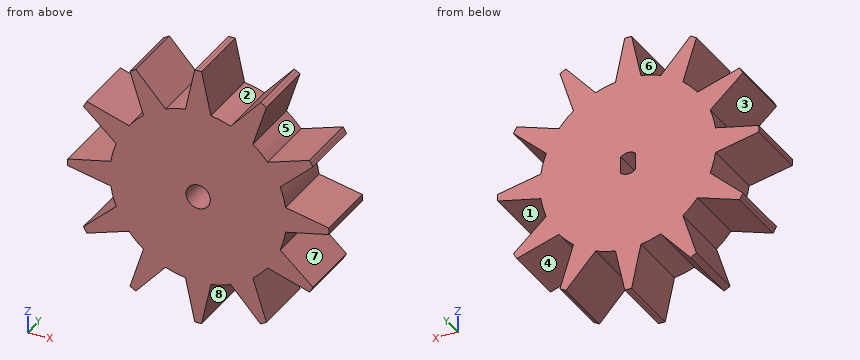
from build123d import *

# Parameters (mm, degrees)
F1_DEPTH = 17.5
F3_DEPTH = 9
F4_R     = 3.25
F5_DEPTH = 9


with BuildPart() as f1:
    # F0 (on Front) → F1 (new body)
    with BuildSketch(Plane.XZ):
        with BuildLine():
            ThreePointArc((23.401412, -3.42), (23.587771, -1.714511), (23.65, 0))
            ThreePointArc((23.65, 0), (23.587771, 1.714511), (23.401412, 3.42))
            ThreePointArc((23.401412, 3.42), (22.844146, 6.12107), (21.976218, 8.738899))
            ThreePointArc((21.976218, 8.738899), (20.481501, 11.825), (18.556218, 14.662513))
            ThreePointArc((18.556218, 14.662513), (16.723075, 16.723075), (14.662513, 18.556218))
            ThreePointArc((14.662513, 18.556218), (11.825, 20.481501), (8.738899, 21.976218))
            ThreePointArc((8.738899, 21.976218), (6.12107, 22.844146), (3.42, 23.401412))
            ThreePointArc((3.42, 23.401412), (0, 23.65), (-3.42, 23.401412))
            ThreePointArc((-3.42, 23.401412), (-6.12107, 22.844146), (-8.738899, 21.976218))
            ThreePointArc((-8.738899, 21.976218), (-11.825, 20.481501), (-14.662513, 18.556218))
            ThreePointArc((-14.662513, 18.556218), (-16.723075, 16.723075), (-18.556218, 14.662513))
            ThreePointArc((-18.556218, 14.662513), (-20.481501, 11.825), (-21.976218, 8.738899))
            ThreePointArc((-21.976218, 8.738899), (-22.844146, 6.12107), (-23.401412, 3.42))
            ThreePointArc((-23.401412, 3.42), (-23.65, 0), (-23.401412, -3.42))
            ThreePointArc((-23.401412, -3.42), (-22.844146, -6.12107), (-21.976218, -8.738899))
            ThreePointArc((-21.976218, -8.738899), (-20.481501, -11.825), (-18.556218, -14.662513))
            ThreePointArc((-18.556218, -14.662513), (-16.723075, -16.723075), (-14.662513, -18.556218))
            ThreePointArc((-14.662513, -18.556218), (-11.825, -20.481501), (-8.738899, -21.976218))
            ThreePointArc((-8.738899, -21.976218), (-6.12107, -22.844146), (-3.42, -23.401412))
            ThreePointArc((-3.42, -23.401412), (0, -23.65), (3.42, -23.401412))
            ThreePointArc((3.42, -23.401412), (6.12107, -22.844146), (8.738899, -21.976218))
            ThreePointArc((8.738899, -21.976218), (11.825, -20.481501), (14.662513, -18.556218))
            ThreePointArc((14.662513, -18.556218), (16.723075, -16.723075), (18.556218, -14.662513))
            ThreePointArc((18.556218, -14.662513), (20.481501, -11.825), (21.976218, -8.738899))
            ThreePointArc((21.976218, -8.738899), (22.844146, -6.12107), (23.401412, -3.42))
        make_face()
        with BuildLine():
            ThreePointArc((23.401412, 3.42), (23.587771, 1.714511), (23.65, 0))
            ThreePointArc((23.65, 0), (23.587771, -1.714511), (23.401412, -3.42))
            Line((23.401412, -3.42), (34.98804, -0.914922))
            Line((34.98804, -0.914922), (35, 0))
            Line((35, 0), (34.98804, 0.914922))
            Line((34.98804, 0.914922), (23.401412, 3.42))
        make_face()
        with BuildLine():
            ThreePointArc((18.556218, 14.662513), (20.481501, 11.825), (21.976218, 8.738899))
            Line((21.976218, 8.738899), (30.757992, 16.701674))
            Line((30.757992, 16.701674), (30.310889, 17.5))
            Line((30.310889, 17.5), (29.84307, 18.286365))
            Line((29.84307, 18.286365), (18.556218, 14.662513))
        make_face()
        with BuildLine():
            Line((30.757992, -16.701674), (21.976218, -8.738899))
            ThreePointArc((21.976218, -8.738899), (20.481501, -11.825), (18.556218, -14.662513))
            Line((18.556218, -14.662513), (29.84307, -18.286365))
            Line((29.84307, -18.286365), (30.310889, -17.5))
            Line((30.310889, -17.5), (30.757992, -16.701674))
        make_face()
        with BuildLine():
            ThreePointArc((8.738899, 21.976218), (11.825, 20.481501), (14.662513, 18.556218))
            Line((14.662513, 18.556218), (18.286365, 29.84307))
            Line((18.286365, 29.84307), (17.5, 30.310889))
            Line((17.5, 30.310889), (16.701674, 30.757992))
            Line((16.701674, 30.757992), (8.738899, 21.976218))
        make_face()
        with BuildLine():
            Line((18.286365, -29.84307), (14.662513, -18.556218))
            ThreePointArc((14.662513, -18.556218), (11.825, -20.481501), (8.738899, -21.976218))
            Line((8.738899, -21.976218), (16.701674, -30.757992))
            Line((16.701674, -30.757992), (17.5, -30.310889))
            Line((17.5, -30.310889), (18.286365, -29.84307))
        make_face()
        with BuildLine():
            ThreePointArc((-3.42, 23.401412), (0, 23.65), (3.42, 23.401412))
            Line((3.42, 23.401412), (0.914922, 34.98804))
            Line((0.914922, 34.98804), (0, 35))
            Line((0, 35), (-0.914922, 34.98804))
            Line((-0.914922, 34.98804), (-3.42, 23.401412))
        make_face()
        with BuildLine():
            Line((0.914922, -34.98804), (3.42, -23.401412))
            ThreePointArc((3.42, -23.401412), (0, -23.65), (-3.42, -23.401412))
            Line((-3.42, -23.401412), (-0.914922, -34.98804))
            Line((-0.914922, -34.98804), (0, -35))
            Line((0, -35), (0.914922, -34.98804))
        make_face()
        with BuildLine():
            ThreePointArc((-14.662513, 18.556218), (-11.825, 20.481501), (-8.738899, 21.976218))
            Line((-8.738899, 21.976218), (-16.701674, 30.757992))
            Line((-16.701674, 30.757992), (-17.5, 30.310889))
            Line((-17.5, 30.310889), (-18.286365, 29.84307))
            Line((-18.286365, 29.84307), (-14.662513, 18.556218))
        make_face()
        with BuildLine():
            Line((-16.701674, -30.757992), (-8.738899, -21.976218))
            ThreePointArc((-8.738899, -21.976218), (-11.825, -20.481501), (-14.662513, -18.556218))
            Line((-14.662513, -18.556218), (-18.286365, -29.84307))
            Line((-18.286365, -29.84307), (-17.5, -30.310889))
            Line((-17.5, -30.310889), (-16.701674, -30.757992))
        make_face()
        with BuildLine():
            ThreePointArc((-21.976218, 8.738899), (-20.481501, 11.825), (-18.556218, 14.662513))
            Line((-18.556218, 14.662513), (-29.84307, 18.286365))
            Line((-29.84307, 18.286365), (-30.310889, 17.5))
            Line((-30.310889, 17.5), (-30.757992, 16.701674))
            Line((-30.757992, 16.701674), (-21.976218, 8.738899))
        make_face()
        with BuildLine():
            Line((-29.84307, -18.286365), (-18.556218, -14.662513))
            ThreePointArc((-18.556218, -14.662513), (-20.481501, -11.825), (-21.976218, -8.738899))
            Line((-21.976218, -8.738899), (-30.757992, -16.701674))
            Line((-30.757992, -16.701674), (-30.310889, -17.5))
            Line((-30.310889, -17.5), (-29.84307, -18.286365))
        make_face()
        with BuildLine():
            ThreePointArc((-23.401412, -3.42), (-23.65, 0), (-23.401412, 3.42))
            Line((-23.401412, 3.42), (-34.98804, 0.914922))
            Line((-34.98804, 0.914922), (-35, 0))
            Line((-35, 0), (-34.98804, -0.914922))
            Line((-34.98804, -0.914922), (-23.401412, -3.42))
        make_face()
    extrude(amount=F1_DEPTH)

    # F2 (on face) → F3 (cut)
    with BuildSketch(Plane(origin=(0, 0, 0), x_dir=(-1, 0, 0), z_dir=(0, 1, 0))):
        with BuildLine():
            Line((2, -2.236068), (2, 2.236068))
            ThreePointArc((2, 2.236068), (0, 3), (-2, 2.236068))
            Line((-2, 2.236068), (-2, -2.236068))
            ThreePointArc((-2, -2.236068), (0, -3), (2, -2.236068))
        make_face()
    extrude(amount=-F3_DEPTH, mode=Mode.SUBTRACT)

    # F4 (on face) → F5 (cut)
    with BuildSketch(Plane.XZ.offset(17.5)):
        Circle(F4_R)
    extrude(amount=-F5_DEPTH, mode=Mode.SUBTRACT)


solid = f1.part
Read the model definition and answer for the solid it produces. Units are mm, in the model's axes. Face numbers are marked on the shaded views. A direction names the side the tool comes from. Give positions to 0.01 mm unless a question says otherwise; leave off trailing zeros. Loops run counter-clockwise (first coordinate to the right, second up) from the corner with the lowest first, then second, coordinate; pieces in that order, holes last. Notation, with made-up numbers: (-0.75, 31.25) -> (45.25, 31.25) arc R14 cw to (45.25, 35.25) -> close; hole circle Ø1 at (56, 12). An arc over 180 degrees is marked (long way). Use a Markdown table: item, result.
Q1. Each of these flat-tipped pins is pushed along its axis until it touches: pin 1 (5 mm diameter, centred on y = -12, z = 20.5, fed in from +X); pin 2 (8 mm diameter, centred on x = -26.5, y = -6.5, fed in from -Z); pin 3 (6 mm diameter, centred on x = -10, y = -8.5, fed in from -Z). Where does it stop, or does it pass through?
Solved:
| item | result |
|---|---|
| pin 1 | stops at x = 30.01 |
| pin 2 | stops at z = -18.29 |
| pin 3 | stops at z = -26.68 |
Q2. Section A-A, the plane z = 28 is taken. Determine the outline of the cut face in (x, y).
Solved:
| item | result |
|---|---|
| outline | (-17.69, -17.5) -> (-14.2, -17.5) -> (-14.2, 0) -> (-17.69, 0) -> close; (-2.43, -17.5) -> (2.43, -17.5) -> (2.43, 0) -> (-2.43, 0) -> close; (14.2, -17.5) -> (17.69, -17.5) -> (17.69, 0) -> (14.2, 0) -> close |
Q3. Determine the mould class of the marked faces 6, 7 and 8 for opening direction Z: pulls with the +Z half, pulls with the -Z half, needs draft (parallel to the pull), parting line crosses it, or undercut.
Solved:
| item | result |
|---|---|
| face 6 | pulls with the +Z half |
| face 7 | undercut |
| face 8 | pulls with the -Z half |
Q4. Section B-B, the plane z = -10.5 is taken. Determine the outline of the cut face in (x, y), then the cut area to 3 significant figures.
Solved:
| item | result |
|---|---|
| outline | (-23.92, -17.5) -> (23.92, -17.5) -> (23.92, 0) -> (-23.92, 0) -> close |
| area | 837 mm^2 |
Q5. Find the intervals of material crossed by line 1 along Z through (x, y) = (0, -10.75); line 2 along X through (y, z) = (-16, 29); line 3 along Z through (x, y) = (-30.5, -7.5), in increasing order.
Solved:
| item | result |
|---|---|
| line 1 | z = -35 to -3.25, 3.25 to 35 |
| line 2 | x = -18.02 to -15.11, -2.21 to 2.21, 15.11 to 18.02 |
| line 3 | z = -17.16 to -16.47, -1.89 to 1.89, 16.47 to 17.16 |
Q6. A tool of negligible diameter and unlimited length cuts with its end or side. For the marked faces 1, 2, 3, 4 and 5, from which of +Z, -Z, +X, -X, +Y, -Y can it reach the whole face along a straight path? Write none if from no direction.
Solved:
| item | result |
|---|---|
| face 1 | +X, +Y, -Y |
| face 2 | +Z, +Y, -Y |
| face 3 | -X, +Y, -Y |
| face 4 | -Z, +Y, -Y |
| face 5 | +Y, -Y |
Q7. Section C-C, the plane z = -21 is taken. Determine the outline of the cut face in (x, y), then the cut area to 3 significant figures.
Solved:
| item | result |
|---|---|
| outline | (-15.45, -17.5) -> (15.45, -17.5) -> (15.45, 0) -> (-15.45, 0) -> close |
| area | 541 mm^2 |
